Work out the finished part from the listing and answer in its coordinate system (mm). Face numbers are marked on the shaded views. A direction names the side the tool comes from. Round coordinates to 2 decimals unless told otherwise and drop trailing zeros. Write each loop counter-clockwise with the first axis right and the second up, starting at its lowest first coordinate (ties: lowest second). Pieces come first, ordered by that corner, then holes.
1. Find section B-B (y = 23). Write down the section's boundary in (x, z).
2. Flat-ended cylindrical pins translate along their axes: pin 1 Ø1 at (x, y) = (11, 18.5) entering from +Z; pin 2 Ø15.5 at (x, z) = (9, 28) entering from -Y; pin 3 Ø8 at (x, y) = (30.5, 22) entering from +Z. Find the tip coordinate at first contact, or state that the pin passes through.
3. Straight lines are drawn through the part: probe 1 along Y at (x, z) = (35, 13); probe 2 along Y at (x, z) = (15, 32). For each, find the intervals that lie inside material, in ascending order.
4. Find section C-C (x = 14). Write down the section's boundary in (y, z), and give its area (3 significant figures).
5. A tool of negligible diameter and unlimited length cuts with its end or side. For the marked faces 1, 2 and 3, from which of +Z, -Z, +X, -X, +Y, -Y can it reach the whole face along a straight path? Write none if from no direction.
6. Find section D-D (z = 12). Write down the section's boundary in (x, y).
7. Find section A-A (z = 34). Write down the section's boundary in (x, y), and give its area (3 significant figures).
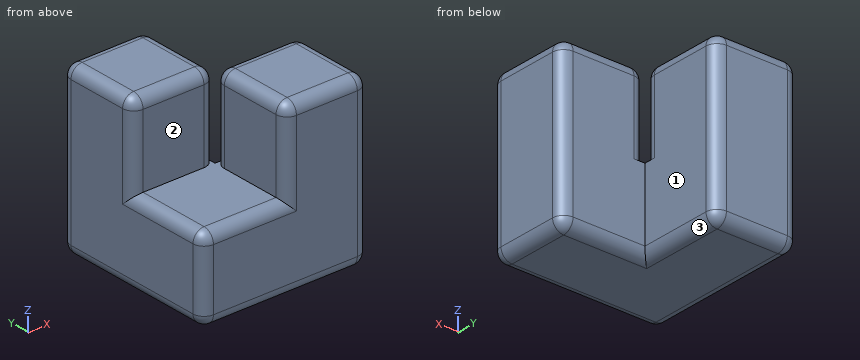
```python
from build123d import *

# Parameters (mm, degrees)
F1_DEPTH = 19.05
F2_W     = 19.05
F2_H     = 19.05
F3_DEPTH = 19.05
F4_R     = 2.54
F5_DEPTH = 19.05
F6_R     = 2.54


with BuildPart() as f1:
    # F0 (on Top) → F1 (new body)
    with BuildSketch(Plane.XY):
        Polygon((0, 38.1), (0, 0), (38.1, 0), (38.1, 19.05), (19.05, 19.05), (19.05, 38.1), align=None)
    extrude(amount=F1_DEPTH)

    # F2 (on face) → F3 (join)
    with BuildSketch(Plane.XY.offset(19.05)):
        with Locations((28.575, 9.525)):
            Rectangle(F2_W, F2_H)
    extrude(amount=F3_DEPTH)

    # F4
    f4_edges = [f1.edges().sort_by_distance(p)[0] for p in [
        (19.05, 19.05, 28.575),
    ]]
    fillet(f4_edges, radius=F4_R)

    # F2 (on face) → F5 (join)
    with BuildSketch(Plane.XY.offset(19.05)):
        with Locations((9.525, 28.575)):
            Rectangle(F2_W, F2_H)
    extrude(amount=F5_DEPTH)

    # F6
    f6_edges = [f1.edges().sort_by_distance(p)[0] for p in [
        (38.1, 0, 19.05),
        (38.1, 9.525, 38.1),
        (38.1, 19.05, 19.05),
        (38.1, 9.525, 0),
        (19.05, 38.1, 19.05),
        (9.525, 38.1, 38.1),
        (0, 38.1, 19.05),
        (9.525, 38.1, 0),
        (0, 28.575, 38.1),
        (9.525, 19.05, 38.1),
        (19.05, 28.575, 38.1),
        (29.845, 19.05, 38.1),
        (19.793949, 18.306051, 38.1),
        (19.05, 8.255, 38.1),
        (28.575, 0, 38.1),
        (0, 19.05, 28.575),
        (0, 9.525, 19.05),
        (0, 0, 9.525),
        (0, 19.05, 0),
        (9.525, 0, 19.05),
        (19.05, 0, 28.575),
        (19.05, 0, 0),
        (28.575, 19.05, 0),
        (19.05, 28.575, 0),
        (19.05, 19.05, 28.575),
    ]]
    fillet(f6_edges, radius=F6_R)


solid = f1.part
```
Worked answers:
1. outline: (0, 2.54) arc R2.54 ccw to (2.54, 0) - (16.51, 0) arc R2.54 ccw to (19.05, 2.54) - (19.05, 35.56) arc R2.54 ccw to (16.51, 38.1) - (2.54, 38.1) arc R2.54 ccw to (0, 35.56) - close
2. pin 1: stops at z = 19.05
2. pin 2: stops at y = 19.05
2. pin 3: stops at z = 37.62
3. probe 1: y = 0 to 19.05
3. probe 2: y = 19.05 to 38.1
4. outline: (0, 2.54) arc R2.54 ccw to (2.54, 0) - (35.56, 0) arc R2.54 ccw to (38.1, 2.54) - (38.1, 35.56) arc R2.54 ccw to (35.56, 38.1) - (21.59, 38.1) arc R2.54 ccw to (19.05, 35.56) - (19.05, 19.05) - (2.54, 19.05) arc R2.54 ccw to (0, 16.51) - close
4. area: 1,080 mm2
5. face 1: +Z, -Z, +X, +Y
5. face 2: +Z, -X, -Y
5. face 3: -Z, +X, +Y
6. outline: (0, 2.54) arc R2.54 ccw to (2.54, 0) - (35.56, 0) arc R2.54 ccw to (38.1, 2.54) - (38.1, 16.51) arc R2.54 ccw to (35.56, 19.05) - (19.05, 19.05) - (19.05, 35.56) arc R2.54 ccw to (16.51, 38.1) - (2.54, 38.1) arc R2.54 ccw to (0, 35.56) - close
7. outline: (0, 21.59) arc R2.54 ccw to (2.54, 19.05) - (16.51, 19.05) arc R2.54 ccw to (19.05, 21.59) - (19.05, 35.56) arc R2.54 ccw to (16.51, 38.1) - (2.54, 38.1) arc R2.54 ccw to (0, 35.56) - close; (19.05, 2.54) arc R2.54 ccw to (21.59, 0) - (35.56, 0) arc R2.54 ccw to (38.1, 2.54) - (38.1, 16.51) arc R2.54 ccw to (35.56, 19.05) - (21.59, 19.05) arc R2.54 ccw to (19.05, 16.51) - close
7. area: 715 mm2
